from build123d import *

# Parameters (mm, degrees)
BOSS_EXTRUDE1_REACH            = 59.868
SKETCH2_W                      = 5
SKETCH2_H                      = 10
SKETCH3_R                      = 4
BOSS_EXTRUDE2_DEPTH            = 1
SKETCH4_R                      = 5.5
BOSS_EXTRUDE3_DEPTH            = 3.5
SKETCH5_R                      = 2.5
BOSS_EXTRUDE4_DEPTH            = 16.5
F_2_5_2_5_DIAMETER_HOLE1_D     = 2.5
F_2_5_2_5_DIAMETER_HOLE1_DEPTH = 28
F_2_5_2_5_DIAMETER_HOLE1_TIP   = 0.751075774
F_3_0_3_DIAMETER_HOLE1_D       = 3
F_3_0_3_DIAMETER_HOLE1_DEPTH   = 28
F_3_0_3_DIAMETER_HOLE1_TIP     = 0.901290929
CHAMFER1_SIZE                  = 1.5
CHAMFER1_SIZE2                 = 4


with BuildPart() as part:
    # Sketch1 → Revolve1 (revolve)
    with BuildSketch(Plane.XY, mode=Mode.PRIVATE) as revolve1_sk:
        Polygon((0, 15.5), (0, 0), (38.5, 0), (38.5, 17.5), (8.5, 17.5), (8.5, 12.5), (7.5, 12.5), (7.5, 17.5), align=None)
    revolve(revolve1_sk.sketch.rotate(Axis((0, 0, 0), (1, 0, 0)), 270), axis=Axis((0, 0, 0), (1, 0, 0)))

    # Sketch2 → Boss-Extrude1 (add, up to next)
    with BuildSketch(Plane.XY.offset(22), mode=Mode.PRIVATE) as boss_extrude1_sk1:
        with Locations((4, 0)):
            Rectangle(SKETCH2_W, SKETCH2_H)
    boss_extrude1_tool1 = extrude(boss_extrude1_sk1.sketch, amount=-BOSS_EXTRUDE1_REACH, mode=Mode.PRIVATE) - part.part
    add(boss_extrude1_tool1.solids().sort_by_distance((4, 0, 22))[0])

    # Sketch3 → Boss-Extrude2 (add)
    with BuildSketch(Plane.ZY):
        Circle(SKETCH3_R)
    extrude(amount=BOSS_EXTRUDE2_DEPTH)

    # Sketch4 → Boss-Extrude3 (add)
    with BuildSketch(Plane(origin=(38.5, 0, 0), x_dir=(0, 0, -1), z_dir=(1, 0, 0))):
        with Locations(Location((0, 0, 0), (0, 0, 180))):
            Circle(SKETCH4_R)
    extrude(amount=BOSS_EXTRUDE3_DEPTH)

    # Sketch5 → Boss-Extrude4 (add)
    with BuildSketch(Plane(origin=(42, 0, 0), x_dir=(0, 0, -1), z_dir=(1, 0, 0))):
        Circle(SKETCH5_R)
    extrude(amount=BOSS_EXTRUDE4_DEPTH)

    # Ø2.5 (2.5) Diameter Hole1
    with Locations(Plane(origin=(38.5, 0, 0), x_dir=(0, 0, -1), z_dir=(1, 0, 0))):
        with Locations((4, -6.92820323), (4, 6.92820323), (-8, 0)):
            Hole(F_2_5_2_5_DIAMETER_HOLE1_D / 2, depth=F_2_5_2_5_DIAMETER_HOLE1_DEPTH)
            with Locations((0, 0, -(F_2_5_2_5_DIAMETER_HOLE1_DEPTH + F_2_5_2_5_DIAMETER_HOLE1_TIP / 2))):  # 118° drill point
                Cone(0, F_2_5_2_5_DIAMETER_HOLE1_D / 2, F_2_5_2_5_DIAMETER_HOLE1_TIP, mode=Mode.SUBTRACT)

    # Ø3.0 (3) Diameter Hole1
    with Locations(Plane.ZY):
        with Locations((-6.717514421, -6.717514421), (8.838834765, -8.838834765), (6.717514421, 6.717514421), (-8.838834765, 8.838834765)):
            Hole(F_3_0_3_DIAMETER_HOLE1_D / 2, depth=F_3_0_3_DIAMETER_HOLE1_DEPTH)
            with Locations((0, 0, -(F_3_0_3_DIAMETER_HOLE1_DEPTH + F_3_0_3_DIAMETER_HOLE1_TIP / 2))):  # 118° drill point
                Cone(0, F_3_0_3_DIAMETER_HOLE1_D / 2, F_3_0_3_DIAMETER_HOLE1_TIP, mode=Mode.SUBTRACT)

    # Chamfer1
    chamfer1_edges = [part.edges().sort_by_distance(p)[0] for p in [
        (38.5, 0, 17.5),
    ]]
    chamfer1_side = [part.faces().sort_by_distance(p)[0] for p in [
        (38.5, 0, 17.005025253),
    ]]
    chamfer(chamfer1_edges, length=CHAMFER1_SIZE, length2=CHAMFER1_SIZE2, reference=chamfer1_side[0])


solid = part.part
For this review, take the finished solid that the model builds, in its own axes (mm). A direction names the side the tool comes from. Round coordinates to 2 decimals unless told otherwise and drop trailing zeros. Loops run counter-clockwise (first coordinate to the right, second up) from the corner with the lowest first, then second, coordinate; pieces in that order, holes last. Notation, with made-up numbers: (34.5, 28) - (59.5, 28) arc R21 cw to (59.5, 33) - close; hole circle Ø7 at (-14, 15.5). An arc over 180 degrees is marked (long way). One line per question, with ' | ' between items.
Q1. The part is to be moulded in two halves that separate along Z. For faces 1 (the conical face through (28.745, 8.68, -9.046)), 2 (the cylindrical face through (50.13, -2.44, 0.54)), 3 (the flat face through (4, 0, 22)), say which applies: released by +Z, released by -Z, zero draft, split by the parting line, or undercut.
Taken from the geometry:
face 1: undercut | face 2: split by the parting line | face 3: released by +Z
Q2. Take a section at C-C (x = 39.5). Give the boundary of the cut face in (y, z).
Taken from the geometry:
outline: circle Ø11 at (0, 0)
Q3. Tool access review of faces 4 (the flat face through (38.5, -7, 0)), 5 (the flat face through (8.5, -8, -11)), 6 (the flat face through (4, 5, 19)): name each direction out of +Z, -Z, +X, -X, +Y, -Y from which nothing blocks a thin tool from reaching the whole face with its end or side.
Taken from the geometry:
face 4: +X | face 5: none | face 6: +Z, -X, +Y
Q4. Take a section at D-D (x = 51.5). Give the boundary of the cut face in (y, z).
Taken from the geometry:
outline: circle Ø5 at (0, 0)
Q5. Take a section at B-B (x = 17). Give the boundary of the cut face in (y, z).
Taken from the geometry:
outline: circle Ø35 at (0, 0); hole circle Ø3 at (-8.84, 8.84); hole (-7.01, -5.25) arc R1.5 ccw (long way) to (-6.65, -5.22) arc R1.25 ccw (long way) to start; hole circle Ø2.5 at (0, 8); hole circle Ø3 at (6.72, 6.72); hole circle Ø2.5 at (6.93, -4); hole circle Ø3 at (8.84, -8.84)
Q6. For pin 1 (2.5 mm diameter, centred on x = 4.5, z = 18, fed in from -Y); pin 2 (3.5 mm diameter, centred on y = -1, z = 17, fed in from -X); pin 3 (1.5 mm diameter, centred on y = 6.93, z = -4, fed in from +X); pin 4 (8 mm diameter, centred on x = 7.5, y = 7, fed in from +Z), all flat-tipped, find the tip position at first contact; note any pin that passes through.
Taken from the geometry:
pin 1: stops at y = -5 | pin 2: stops at x = 0 | pin 3: stops at x = 10.2 | pin 4: stops at z = 22
Q7. Take a section at A-A (z = 0). Give the boundary of the cut face in (x, y), and give its area (3 significant figures).
Taken from the geometry:
outline: (-1, -4) - (0, -4) - (0, -15.5) - (7.5, -17.5) - (7.5, -12.5) - (8.5, -12.5) - (8.5, -17.5) - (34.5, -17.5) - (38.5, -16) - (38.5, -5.5) - (42, -5.5) - (42, -2.5) - (58.5, -2.5) - (58.5, 2.5) - (42, 2.5) - (42, 5.5) - (38.5, 5.5) - (38.5, 16) - (34.5, 17.5) - (8.5, 17.5) - (8.5, 12.5) - (7.5, 12.5) - (7.5, 17.5) - (0, 15.5) - (0, 4) - (-1, 4) - close | area: 1,450 mm²
Q8. For line 1 along X through (y, z) = (-1.5, 12.5); line 2 along Y through (x, z) = (24.75, 8); line 3 along X through (y, z) = (-4, -9), list the stretches that pass through material, from the lowest coordinate up. Write a range as [from, to].
Taken from the geometry:
line 1: x = [0, 7.5], [8.5, 38.5] | line 2: y = [-15.56, -10.08], [-7.6, -1.25], [1.25, 5.94], [7.5, 15.56] | line 3: x = [0, 38.5]
